```python
from build123d import *

# Parameters (mm, degrees)
SKETCH1_W           = 49.8113264
SKETCH1_H           = 241.325
SKETCH1_W_2         = 5
SKETCH1_H_2         = 6.35
SKETCH1_W_3         = 25
BOSS_EXTRUDE1_DEPTH = 6.35
BOSS_EXTRUDE2_DEPTH = 6.35


with BuildPart() as part:
    # Sketch1 → Boss-Extrude1 (new body)
    with BuildSketch(Plane.XY):
        Rectangle(SKETCH1_W, SKETCH1_H)
        with Locations((17.4056632, 123.8375)):
            Rectangle(SKETCH1_W_2, SKETCH1_H_2)
        with Locations((7.4056632, 123.8375)):
            Rectangle(SKETCH1_W_2, SKETCH1_H_2)
        with Locations((7.4056632, -123.8375)):
            Rectangle(SKETCH1_W_2, SKETCH1_H_2)
        with Locations((17.4056632, -123.8375)):
            Rectangle(SKETCH1_W_2, SKETCH1_H_2)
        with Locations((37.4056632, 0)):
            Rectangle(SKETCH1_W_3, SKETCH1_H)
    extrude(amount=BOSS_EXTRUDE1_DEPTH)

    # Sketch2 → Boss-Extrude2 (add)
    with BuildSketch(Plane.XY.offset(6.35)):
        Polygon((49.9463032, -120.70314), (49.9463032, 120.70314), (19.9463032, 120.70314), (19.9463032, 127.05314), (14.8650232, 127.05314), (14.8650232, 120.70314), (9.9463032, 120.70314), (9.9463032, 127.05314), (4.8650232, 127.05314), (4.8650232, 120.70314), (-24.9463032, 120.70314), (-24.9463032, -120.70314), (4.8650232, -120.70314), (4.8650232, -127.05314), (9.9463032, -127.05314), (9.9463032, -120.70314), (14.8650232, -120.70314), (14.8650232, -127.05314), (19.9463032, -127.05314), (19.9463032, -120.70314), align=None)
    extrude(amount=-BOSS_EXTRUDE2_DEPTH)


solid = part.part
```
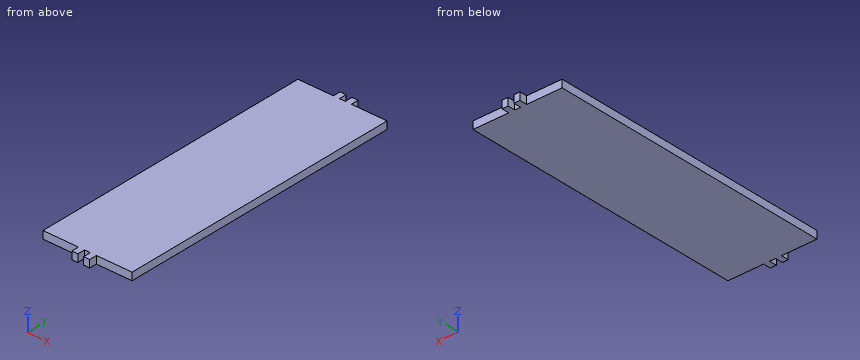
Can you work these out from the model? Positions are in its coordinate system, mm. Coordinates: 2 decimals unless noted, no trailing zeros. Loops run counter-clockwise (first coordinate to the right, second up) from the corner with the lowest first, then second, coordinate; pieces in that order, holes last. Notation, with made-up numbers: (-13.5, -22.5) - (44.5, -22.5) arc R11 cw to (44.5, -3.5) - close; hole circle Ø8 at (37, 87.5). An arc over 180 degrees is marked (long way). Answer as CSV lines item,"result". Start each with the question number.
1) Suppose I cut it at A-A (z = 3). Please give me the cut outline in (x, y), plus the area to 3 significant figures.
2) I need wall thicknesses on line 1 (Y direction, x = 20, z = 5.75). Which ranges of the line are inside material? Lowest first, please. Write a range as from..to.
3) For pin 1 (1 mm diameter, centred on x = 40.5, z = 1, fed in from +Y); pin 2 (2.5 mm diameter, centred on x = 11.5, z = 4.5, fed in from -Y); pin 3 (1.9 mm diameter, centred on y = 123.5, z = 4.5, fed in from -X) (3 decimals), each with a flat end and sliding along its axis, tell me the tip position at first contact or that it passes through.
4) Suppose I cut it at B-B (x = -7.5). Please give me the cut outline in (y, z), plus the area to 3 significant figures.
Check result:
1,outline,"(-24.95, -120.7) - (4.87, -120.7) - (4.87, -127.05) - (9.95, -127.05) - (9.95, -120.7) - (14.87, -120.7) - (14.87, -127.05) - (19.95, -127.05) - (19.95, -120.7) - (49.95, -120.7) - (49.95, 120.7) - (19.95, 120.7) - (19.95, 127.05) - (14.87, 127.05) - (14.87, 120.7) - (9.95, 120.7) - (9.95, 127.05) - (4.87, 127.05) - (4.87, 120.7) - (-24.95, 120.7) - close"
1,area,"18,200 mm²"
2,line 1,"y = -120.7..120.7"
3,pin 1,"stops at y = 120.7"
3,pin 2,"stops at y = -120.7"
3,pin 3,"stops at x = 4.865"
4,outline,"(-120.7, 0) - (120.7, 0) - (120.7, 6.35) - (-120.7, 6.35) - close"
4,area,"1,530 mm²"
